Check sheet for the modelled part. Datum: model origin and axes. Units: mm. Round coordinates to 2 decimals unless told otherwise and drop trailing zeros. One line per item, written item: value.
Autodesk Fusion 360 part; units mm, degrees
sketch "Sketch1" plane through (0, 0, 0) normal (0, 0, 1) x (1, 0, 0)
  line L0 (0, 0) -> (680, 0)
  line L1 (680, 0) -> (680, -304)
  line L2 (680, -304) -> (0, -304)
  line L3 (0, -304) -> (0, 0)
  dimension "d1" = 680
  dimension "d2" = 304
extrude "Extrude1" add sketch "Sketch1" along normal blind 6.25
sketch "Sketch2" plane through (0, 0, 6.25) normal (0, 0, 1) x (-1, 0, 0)
  line L0 (0, 304) -> (-680, 304)
  line L1 (-680, 304) -> (-680, 0)
  line L2 (-680, 0) -> (0, 0)
  line L3 (0, 0) -> (0, 304)
  line L4 (-160, 120) -> (-160, 167)
  line L5 (-160, 167) -> (0, 167)
  line L6 (0, 167) -> (0, 78)
  line L7 (-120, 78) -> (-120, 120)
  line L8 (-120, 120) -> (-160, 120)
  line L9 (-120, 78) -> (0, 78)
  line L10 (-680, 304) -> (-600, 304)
  line L11 (-600, 304) -> (-600, 194)
  line L12 (-600, 194) -> (-655, 194)
  line L13 (-680, 175) -> (-680, 304)
  line L14 (-655, 194) -> (-680, 175)
  dimension "d10" = 120
  dimension "d11" = 42
  dimension "d12" = 47
  dimension "d13" = 120
  dimension "d14" = 160
  dimension "d15" = 110
  dimension "d19" = 129
  dimension "d20" = 55
  dimension "d21" = 80
extrude "Extrude3" cut sketch "Sketch2" against normal blind 6.25 contours L0 L1 L10 L11 L12 L13 L14 | L3 L4 L5 L6 L7 L8 L9
sketch "Sketch4" plane through (0, 0, 6.25) normal (0, 0, 1) x (-1, 0, 0)
  line L0 (-160, 167) -> (0, 167)
  line L1 (0, 167) -> (0, 304)
  line L2 (0, 304) -> (-600, 304)
  line L3 (-600, 304) -> (-600, 194)
  line L4 (-600, 194) -> (-655, 194)
  line L5 (-655, 194) -> (-680, 175)
  line L6 (-680, 175) -> (-680, 0)
  line L7 (-680, 0) -> (0, 0)
  line L8 (0, 0) -> (0, 78)
  line L9 (0, 78) -> (-120, 78)
  line L10 (-120, 78) -> (-120, 120)
  line L11 (-120, 120) -> (-160, 120)
  line L12 (-160, 120) -> (-160, 167)
  line L13 (-69, 200) -> (-115, 200) construction
  line L14 (-597, 145) -> (-643, 145) construction
  line L15 (-115, 50) -> (-69, 50) construction
  line L16 (-597, 50) -> (-643, 50) construction
  point P0 (-643, 145)
  point P1 (-597, 145)
  point P2 (-115, 200)
  point P3 (-69, 200)
  point P4 (-115, 50)
  point P5 (-69, 50)
  point P6 (-597, 50)
  point P7 (-643, 50)
  dimension "d33" = 46
  dimension "d35" = 150
  dimension "d36" = 50
  dimension "d37" = 95
  dimension "d38" = 115
  dimension "d44" = 83
hole "Hole2" at (597, -145, 6.25) at (643, -145, 6.25) at (115, -200, 6.25) at (69, -200, 6.25) at (115, -50, 6.25) at (69, -50, 6.25) at (643, -50, 6.25) at (597, -50, 6.25) direction (0, 0, -1) diameter 8.5 depth 6.25 tip angle 118
sketch "Sketch5" plane through (0, 0, 6.25) normal (0, 0, 1) x (-1, 0, 0)
  circle A0 centre (-643, 50) radius 4.25
  circle A1 centre (-115, 50) radius 4.25
  circle A2 centre (-115, 200) radius 4.25
  circle A3 centre (-597, 145) radius 4.25
  circle A4 centre (-643, 145) radius 4.25
  circle A5 centre (-69, 200) radius 4.25
  circle A6 centre (-69, 50) radius 4.25
  circle A7 centre (-597, 50) radius 4.25
  line L0 (-160, 167) -> (0, 167)
  line L1 (0, 167) -> (0, 304)
  line L2 (0, 304) -> (-600, 304)
  line L3 (-600, 304) -> (-600, 194)
  line L4 (-600, 194) -> (-655, 194)
  line L5 (-655, 194) -> (-680, 175)
  line L6 (-680, 175) -> (-680, 0)
  line L7 (-680, 0) -> (0, 0)
  line L8 (0, 0) -> (0, 78)
  line L9 (0, 78) -> (-120, 78)
  line L10 (-120, 78) -> (-120, 120)
  line L11 (-120, 120) -> (-160, 120)
  line L12 (-160, 120) -> (-160, 167)
  line L13 (-225, 0) -> (-225, 130) construction
  line L14 (-587, 0) -> (-587, 304) construction
  line L15 (-390, 0) -> (-390, 304) construction
  line L16 (-225, 130) -> (-160, 130) construction
  line L17 (-347.9611, 97.8111) -> (-427.9611, 97.8111) construction
  line L18 (-427.9611, 97.8111) -> (-427.9611, 77.8111) construction
  line L19 (-427.9611, 77.8111) -> (-347.9611, 77.8111) construction
  line L20 (-347.9611, 77.8111) -> (-347.9611, 97.8111) construction
  line L21 (-560, 0) -> (-560, 304) construction
  dimension "d39" = 225
  dimension "d41" = 390
  dimension "d42" = 130
  dimension "d43" = 10
  dimension "d46" = 170
  dimension "d47" = 93
equation "d19 = 304 mm - 175 mm"
Item 1: Sectioned sample at A-A on z = 4.5. Count the separate pieces of the cut face and the enclosed holes in it, and give its area (3 significant figures).
Answer:
separate pieces: 1
enclosed holes: 8
area: 185,000 mm^2
Item 2: Thickness scan on line 1 (Y direction, x = 643, z = 4.25); line 2 (Y direction, x = 69, z = 3.5); line 3 (X direction, y = -200, z = 3.5). Record the ranges inside material, lowest first.
Answer:
line 1: y = -194 to -149.25, -140.75 to -54.25, -45.75 to 0
line 2: y = -304 to -204.25, -195.75 to -167, -78 to -54.25, -45.75 to 0
line 3: x = 0 to 64.75, 73.25 to 110.75, 119.25 to 600
Item 3: Depth check by flat-ended pin: P1, Ø5, axis at x = 643, y = -145, coming from the +Z side; P2, Ø3, axis at y = -135.5, z = 4.5, coming from the -X side. Enter the tip coordinate at first touch or a pass-through.
Answer:
P1: passes through
P2: stops at x = 160
